Could you check a few things on this drawing? It's one solid part, dimensions in mm from its lowest x, y, z. A direction names the side the tool comes from. Give positions to 0.01 mm unless a question says otherwise; leave off trailing zeros. Order: outer loops, then holes, each group sorted by start corner. A loop starts at its lowest first (then second) coordinate and runs counter-clockwise, first axis right, second up.
Item 1: I want a section at C-C, the plane x = 28.5. Write out the boundary of the cut face in (y, z).
Item 2: If I drill on line 1 along X through (y, z) = (2.05, 18); line 2 along X through (y, z) = (5.75, 6.5), over which ranges is the centre line in solid material (lowest first)?
Item 3: Which directions (+Z, -Z, +X, -X, +Y, -Y) give clear straight access to the entire face, cutting with the end or side of a thin tool? Please do the marked faces 1 and 2.
Item 4: I want a section at D-D, the plane z = 5. Write out the boundary of the cut face in (x, y), then the cut area to 3 significant figures.
Item 5: I'm going to push flat-ended pins straight in: pin 1 Ø3.5 at (x, z) = (9.5, 14) entering from +Y; pin 2 Ø1.5 at (x, z) = (18, 22.5) entering from +Y; pin 3 Ø8 at (x, z) = (18, 4.5) entering from +Y. Where does each tip first touch, or does it pass through?
Item 6: If we mould it in two halves opening along X, with no side actions, what happens to the marked faces 3, 4 and 5? For each: +X half, -X half, draft (parallel to the pull), parting line (faces both ways), or undercut.
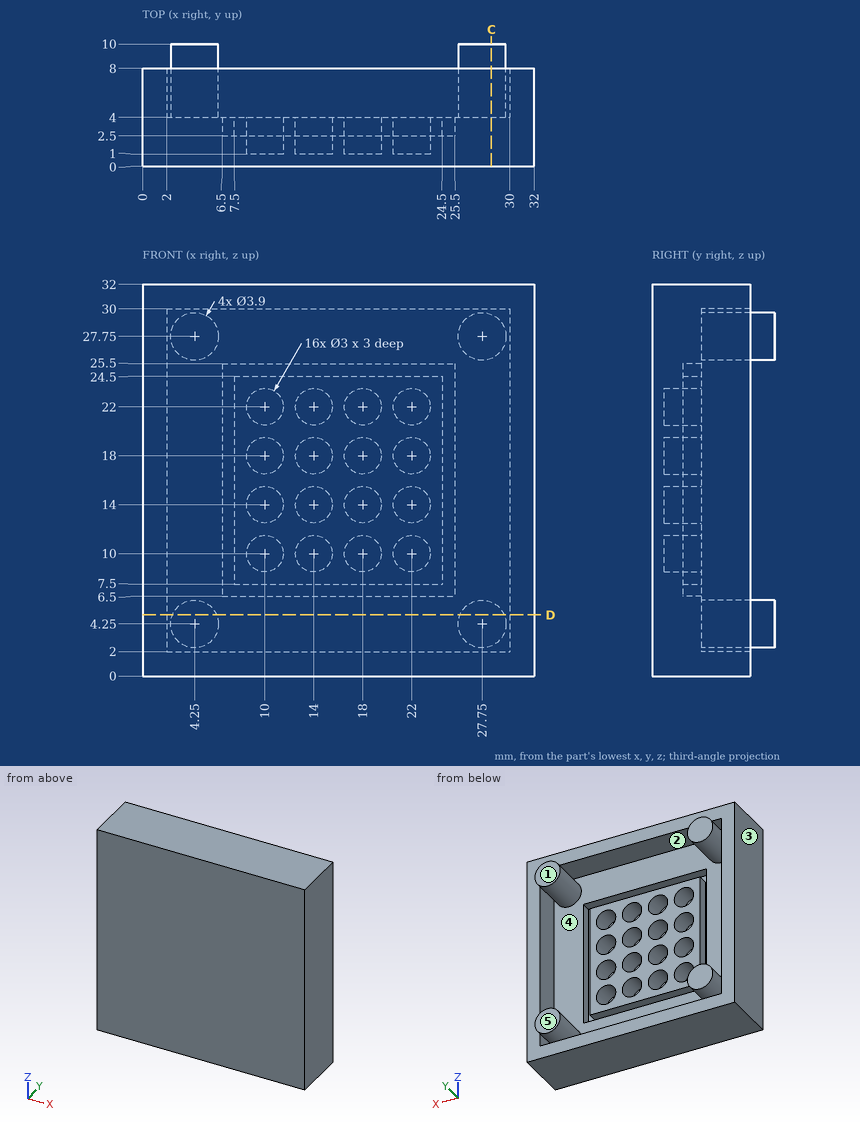
Results list:
1. outline: (0, 0) - (8, 0) - (8, 2) - (4, 2) - (4, 2.45) - (10, 2.45) - (10, 6.05) - (4, 6.05) - (4, 25.95) - (10, 25.95) - (10, 29.55) - (4, 29.55) - (4, 30) - (8, 30) - (8, 32) - (0, 32) - close
2. line 1: x = 0 to 8.5, 11.5 to 12.5, 15.5 to 16.5, 19.5 to 20.5, 23.5 to 32
2. line 2: x = 0 to 2, 30 to 32
3. face 1: +Z, -Z, +X, -X, +Y
3. face 2: +Y
4. outline: (0, 0) - (32, 0) - (32, 8) - (30, 8) - (30, 4) - (29.55, 4) - (29.55, 10) - (25.95, 10) - (25.95, 4) - (6.05, 4) - (6.05, 10) - (2.45, 10) - (2.45, 4) - (2, 4) - (2, 8) - (0, 8) - close
4. area: 187 mm2
5. pin 1: stops at y = 4
5. pin 2: stops at y = 1
5. pin 3: stops at y = 8
6. face 3: -X half
6. face 4: undercut
6. face 5: draft
